Work out the finished part from the listing and answer in its coordinate system (mm). Face numbers are marked on the shaded views. Give positions to 0.01 mm unless a question says otherwise; leave off trailing zeros. Loops run counter-clockwise (first coordinate to the right, second up) from the corner with the lowest first, then second, coordinate; pieces in that order, holes last. Notation, with made-up numbers: M 8,-3.5 L 34,-3.5 A36 cw 34,31.5 Z; hole C -12.5,-10.5 d6. An arc over 180 degrees is marked long. Use a Markdown table: item, result.
```python
from build123d import *

# Parameters (mm, degrees)
SKETCH1_R           = 1.5
BOSS_EXTRUDE1_DEPTH = 3
BOSS_EXTRUDE2_START = 3
SKETCH1_3_W         = 11.8
SKETCH1_3_H         = 1.4
SKETCH1_3_W_2       = 125
SKETCH1_3_H_2       = 2
BOSS_EXTRUDE2_DEPTH = 3.7
SKETCH2_R           = 1.5
CUT_EXTRUDE1_DEPTH  = 69.411548733
SKETCH3_R           = 6
SKETCH3_R_2         = 1.5
BOSS_EXTRUDE3_DEPTH = 0.2


with BuildPart() as part:
    # Sketch1 → Boss-Extrude1 (new body)
    with BuildSketch(Plane(origin=(0, 0, 0), x_dir=(1, 0, 0), z_dir=(0, 1, 0))):
        with BuildLine():
            Line((-62.5, 0), (-5.9, 0))
            Line((-5.9, 0), (-5.9, -1.4))
            Line((-5.9, -1.4), (5.9, -1.4))
            Line((5.9, -1.4), (5.9, 0))
            Line((5.9, 0), (62.5, 0))
            Line((62.5, 0), (62.5, 16.5))
            ThreePointArc((62.5, 16.5), (56.588078143, 27.122957516), (44.444443779, 27.697579876))
            ThreePointArc((44.444443779, 27.697579876), (-1.61e-07, 17.278221854), (-44.444444068, 27.697580019))
            ThreePointArc((-44.444444068, 27.697580019), (-56.58807828, 27.122957431), (-62.5, 16.5))
            Line((-62.5, 16.5), (-62.5, 0))
        make_face()
        with Locations(Location((50, 16.5, 0), (0, 0, 270))):
            Circle(SKETCH1_R, mode=Mode.SUBTRACT)
        with Locations(Location((-50, 16.5, 0), (0, 0, 270))):
            Circle(SKETCH1_R, mode=Mode.SUBTRACT)
    extrude(amount=BOSS_EXTRUDE1_DEPTH)

    # Sketch1<3> → Boss-Extrude2 (add)
    with BuildSketch(Plane(origin=(0, 0, 0), x_dir=(1, 0, 0), z_dir=(0, 1, 0)).offset(BOSS_EXTRUDE2_START)):
        with BuildLine():
            ThreePointArc((-46, 16.5), (-50, 20.5), (-54, 16.5))
            Line((-54, 16.5), (-51.5, 16.5))
            ThreePointArc((-51.5, 16.5), (-50, 18), (-48.5, 16.5))
            Line((-48.5, 16.5), (-46, 16.5))
        make_face()
        with BuildLine():
            Line((-51.5, 16.5), (-54, 16.5))
            ThreePointArc((-54, 16.5), (-50, 12.5), (-46, 16.5))
            Line((-46, 16.5), (-48.5, 16.5))
            ThreePointArc((-48.5, 16.5), (-50, 15), (-51.5, 16.5))
        make_face()
        with BuildLine():
            ThreePointArc((46, 16.5), (50, 12.5), (54, 16.5))
            Line((54, 16.5), (51.5, 16.5))
            ThreePointArc((51.5, 16.5), (50, 15), (48.5, 16.5))
            Line((48.5, 16.5), (46, 16.5))
        make_face()
        with BuildLine():
            Line((51.5, 16.5), (54, 16.5))
            ThreePointArc((54, 16.5), (50, 20.5), (46, 16.5))
            Line((46, 16.5), (48.5, 16.5))
            ThreePointArc((48.5, 16.5), (50, 18), (51.5, 16.5))
        make_face()
        with Locations((0, -0.7)):
            Rectangle(SKETCH1_3_W, SKETCH1_3_H)
        with Locations((0, 1)):
            Rectangle(SKETCH1_3_W_2, SKETCH1_3_H_2)
    extrude(amount=BOSS_EXTRUDE2_DEPTH)

    # Sketch2 → Cut-Extrude1 (cut, through all)
    with BuildSketch(Plane(origin=(0, 0, -2), x_dir=(-1, 0, 0), z_dir=(0, 0, -1))):
        with Locations((0, 6.7)):
            Circle(SKETCH2_R)
    extrude(amount=-CUT_EXTRUDE1_DEPTH, mode=Mode.SUBTRACT)

    # Sketch3 → Boss-Extrude3 (add)
    with BuildSketch(Plane(origin=(0, 3, 0), x_dir=(1, 0, 0), z_dir=(0, 1, 0))):
        with Locations(Location((-50, 16.5, 0), (0, 0, 270))):
            Circle(SKETCH3_R)
        with Locations(Location((-50, 16.5, 0), (0, 0, 270))):
            Circle(SKETCH3_R_2, mode=Mode.SUBTRACT)
        with Locations(Location((50, 16.5, 0), (0, 0, 270))):
            Circle(SKETCH3_R)
        with Locations(Location((50, 16.5, 0), (0, 0, 270))):
            Circle(SKETCH3_R_2, mode=Mode.SUBTRACT)
    extrude(amount=BOSS_EXTRUDE3_DEPTH)


solid = part.part
```
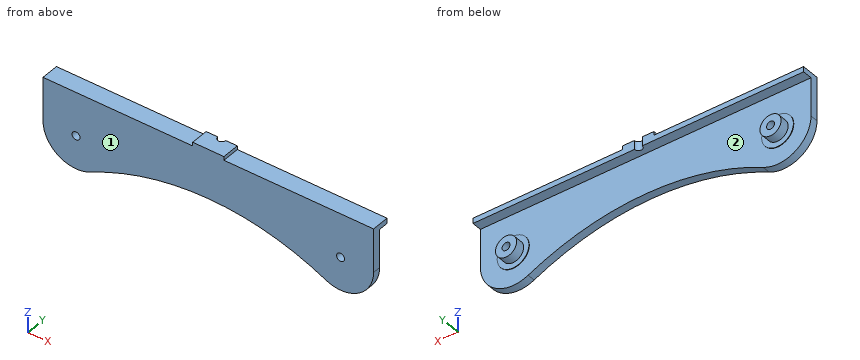
(1) A cutting plane is placed at D-D (x = 32). Write down the section's boundary in (y, z), and give its area (3 significant figures).
Entries:
| item | result |
|---|---|
| outline | M 0,-22.54 L 3,-22.54 L 3,-2 L 6.7,-2 L 6.7,0 L 0,0 Z |
| area | 75.0 mm² |
(2) Given P1, Ø2, axis at x = -30, y = 2.5, coming from the +Z side; P2, Ø2.5, axis at x = -50, z = -16.5, coming from the +Y side; P3, Ø0.7, axis at y = 4.5, z = 0.5, coming from the +X side; P4, Ø6, axis at x = -45, z = -22, coming from the +Y side, each flat-ended and moving along its own axis, determine where each tip first touches the part or whether it passes through.
Entries:
| item | result |
|---|---|
| P1 | stops at z = 0 |
| P2 | passes through |
| P3 | stops at x = 5.9 |
| P4 | stops at y = 3.2 |
(3) The mould has two halves that part along X. Classify the marked faces 1 and 2: released by +X, released by -X, zero draft, split by the parting line, or undercut.
Entries:
| item | result |
|---|---|
| face 1 | zero draft |
| face 2 | undercut |
(4) A cutting plane is placed at B-B (x = 0). Write down the section's boundary in (y, z), and give its area (3 significant figures).
Entries:
| item | result |
|---|---|
| outline | M 0,-17.28 L 3,-17.28 L 3,-2 L 5.2,-2 L 5.2,1.4 L 0,1.4 Z |
| area | 63.5 mm² |
(5) A cutting plane is placed at C-C (z = -6). Write down the section's boundary in (x, y), and give its area (3 significant figures).
Entries:
| item | result |
|---|---|
| outline | M -62.5,0 L 62.5,0 L 62.5,3 L -62.5,3 Z |
| area | 375 mm² |
(6) A cutting plane is placed at A-A (z = -24.5). Write down the section's boundary in (x, y).
Entries:
| item | result |
|---|---|
| outline | M -59.6,0 L -37.31,0 L -37.31,3 L -59.6,3 Z; M 37.31,0 L 59.6,0 L 59.6,3 L 37.31,3 Z |
(7) Consider probe 1 along X at (y, z) = (3.1, -16.5); probe 2 along Z at (x, y) = (-50, 5.7); probe 3 along X at (y, z) = (1.65, -16.5). Determine where each line is inside the solid, lowest interval first. Write a range as [from, to].
Entries:
| item | result |
|---|---|
| probe 1 | x = [-56, -51.5], [-48.5, -44], [44, 48.5], [51.5, 56] |
| probe 2 | z = [-20.5, -18], [-15, -12.5], [-2, 0] |
| probe 3 | x = [-62.5, -51.5], [-48.5, 48.5], [51.5, 62.5] |
